from build123d import *

# Parameters (mm, degrees)
SKETCH1_R                   = 13.21
SKETCH1_R_2                 = 2.1
BOSS_EXTRUDE1_DEPTH         = 20
CHAMFER1_SIZE               = 1.2
BOSS_EXTRUDE5_START         = 40
SKETCH7_R                   = 13.21
SKETCH7_R_2                 = 3.3
BOSS_EXTRUDE5_DEPTH         = 40
CUT_EXTRUDE3_START          = -0.5
SKETCH8_W                   = 13.21
SKETCH8_H                   = 35.8
CUT_EXTRUDE3_DEPTH          = 1
SKETCH11_W                  = 13.21
SKETCH11_H                  = 35.8
CUT_EXTRUDE5_DEPTH          = 2.5
CUT_EXTRUDE6_DEPTH          = 45.29975395
CUT_EXTRUDE6_DEPTH_BACK     = 45.29975395
SKETCH12_R                  = 1.2
SKETCH13_R                  = 2.5
CUT_EXTRUDE7_DEPTH          = 47.093038676
SKETCH15_R                  = 1.8
BOSS_EXTRUDE6_DEPTH         = 5
BOSS_EXTRUDE7_REACH         = 61.49
CIRPATTERN2_COUNT           = 4
CIRPATTERN2_COPY_1_SKETCH_R = 1.8
CIRPATTERN2_COPY_1_DEPTH    = 5
CIRPATTERN2_COPY_2_SKETCH_R = 1.8
CIRPATTERN2_COPY_2_DEPTH    = 5
CIRPATTERN2_COPY_3_SKETCH_R = 1.8
CIRPATTERN2_COPY_3_DEPTH    = 5
CHAMFER2_SIZE               = 6.994614872
CHAMFER2_SIZE2              = 15


with BuildPart() as part:
    # Sketch1 → Boss-Extrude1 (new body)
    with BuildSketch(Plane(origin=(0, 0, 0), x_dir=(1, 0, 0), z_dir=(0, 1, 0))):
        with Locations(Location((0, 0, 0), (0, 0, 270))):
            Circle(SKETCH1_R)
        with Locations(Location((0, 0, 0), (0, 0, 270))):
            Circle(SKETCH1_R_2, mode=Mode.SUBTRACT)
    extrude(amount=BOSS_EXTRUDE1_DEPTH)

    # Chamfer1
    chamfer1_edges = [part.edges().sort_by_distance(p)[0] for p in [
        (0, 0, -2.1),
    ]]
    chamfer(chamfer1_edges, length=CHAMFER1_SIZE)

    # Sketch7 → Boss-Extrude5 (add)
    with BuildSketch(Plane.XZ.offset(BOSS_EXTRUDE5_START)):
        with Locations(Location((0, 0, 0), (0, 0, 270))):
            Circle(SKETCH7_R)
        with Locations(Location((0, 0, 0), (0, 0, 270))):
            Circle(SKETCH7_R_2, mode=Mode.SUBTRACT)
    extrude(amount=-BOSS_EXTRUDE5_DEPTH)

    # Sketch8 → Cut-Extrude3 (cut)
    with BuildSketch(Plane(origin=(0, 0, 0), x_dir=(0, 0, -1), z_dir=(1, 0, 0)).offset(CUT_EXTRUDE3_START)):
        with Locations((-6.605, -22.1)):
            Rectangle(SKETCH8_W, SKETCH8_H)
    extrude(amount=CUT_EXTRUDE3_DEPTH, mode=Mode.SUBTRACT)

    # Sketch11 → Cut-Extrude5 (cut, symmetric)
    with BuildSketch(Plane(origin=(0, 0, 0), x_dir=(0, 0, -1), z_dir=(1, 0, 0))):
        with Locations((6.605, -22.1)):
            Rectangle(SKETCH11_W, SKETCH11_H)
    extrude(amount=CUT_EXTRUDE5_DEPTH, both=True, mode=Mode.SUBTRACT)

    # Sketch12 → Cut-Extrude6 (cut, two sides: drawn at the far end of the back side and taken through both)
    with BuildSketch(Plane.ZY.offset(-0.5).offset(-CUT_EXTRUDE6_DEPTH_BACK)):
        with Locations((10.21, -8.2)):
            Circle(SKETCH12_R)
    extrude(amount=CUT_EXTRUDE6_DEPTH + CUT_EXTRUDE6_DEPTH_BACK, mode=Mode.SUBTRACT)

    # Sketch13 → Cut-Extrude7 (cut, through all)
    with BuildSketch(Plane.ZY.offset(-5.5)):
        with Locations((10.21, -8.2)):
            Circle(SKETCH13_R)
    cut_extrude7 = extrude(amount=-CUT_EXTRUDE7_DEPTH, mode=Mode.SUBTRACT)

    # Mirror2: Cut-Extrude7 across plane
    add(cut_extrude7.mirror(Plane(origin=(0, 0, 0), x_dir=(0, 0, 1), z_dir=(1, 0, 0))), mode=Mode.SUBTRACT)

    # Sketch15 → Boss-Extrude6 (add)
    with BuildSketch(Plane(origin=(-1.060660172, 0, -1.060660172), x_dir=(-0.7071067811865488, -3.372135297382167e-15, 0.7071067811865462), z_dir=(-0.7071067811865462, 3.3721352973821793e-15, -0.7071067811865488))):
        Polygon((-22.70423895, -23.81017386), (-11.21, -23.81017386), (-11.21, -35.211035784), (-11.21, -40), (-15.990174244, -46.657077484), (-29.831605047, -40.876524454), align=None)
        with Locations((-19.21, -29.81017386)):
            Circle(SKETCH15_R, mode=Mode.SUBTRACT)
        with Locations((-19.21, -38.81017386)):
            Circle(SKETCH15_R, mode=Mode.SUBTRACT)
    boss_extrude6 = extrude(amount=BOSS_EXTRUDE6_DEPTH)

    # Mirror3: Boss-Extrude6 across plane
    add(boss_extrude6.mirror(Plane(origin=(0, 0, 0), x_dir=(-0.7071067811865488, 3.3721352973821916e-15, 0.7071067811865464), z_dir=(0.7071067811865462, -3.3721352973821793e-15, 0.7071067811865488))))

    # Boss-Extrude7: up to this face of the body (flat: up to its plane)
    boss_extrude7_end = Plane(part.part.faces().sort_by_distance((18.066702505, -34.728946199, -8.87431435))[0])
    # Sketch16 → Boss-Extrude7 (add, up to the picked face)
    with BuildSketch(Plane(origin=(-4.596194078, 0, -4.596194078), x_dir=(-0.7071067811865486, -3.1363800445660566e-15, 0.7071067811865465), z_dir=(-0.7071067811865465, 3.1363800445660664e-15, -0.7071067811865486)), mode=Mode.PRIVATE) as boss_extrude7_sk1:
        with BuildLine():
            Line((-11.500178259, -23.81017386), (-22.70423895, -23.81017386))
            ThreePointArc((-22.70423895, -23.81017386), (-18.231146382, -18.383887076), (-11.500178259, -16.347416226))
            Line((-11.500178259, -16.347416226), (-11.500178259, -23.81017386))
        make_face()
    boss_extrude7_tool1 = split(extrude(boss_extrude7_sk1.sketch, amount=-BOSS_EXTRUDE7_REACH, mode=Mode.PRIVATE), bisect_by=boss_extrude7_end, keep=Keep.BOTH, mode=Mode.PRIVATE)
    boss_extrude7 = boss_extrude7_tool1.solids().sort_by(Axis((6.682248, -20.729124, -15.874636), (0.7071067811865465, -3.1363800445660664e-15, 0.7071067811865486)))[0]
    add(boss_extrude7)

    # CirPattern2: Boss-Extrude6, Boss-Extrude7 ×4 about axis
    cirpattern2_axis = Axis((0, 0, 0), (0, 1, 0))
    add([boss_extrude6.rotate(cirpattern2_axis, i * 360 / CIRPATTERN2_COUNT) for i in range(1, CIRPATTERN2_COUNT)])
    add([boss_extrude7.rotate(cirpattern2_axis, i * 360 / CIRPATTERN2_COUNT) for i in range(1, CIRPATTERN2_COUNT)])

    # CirPattern2 copy 1 sketch → CirPattern2 copy 1 (add)
    with BuildSketch(Plane(origin=(1.060660172, 0, -1.060660172), x_dir=(0.7071067811865462, -3.372135297382167e-15, 0.7071067811865489), z_dir=(0.7071067811865488, -3.3721352973821793e-15, -0.7071067811865461))):
        Polygon((-22.70423895, 23.81017386), (-11.21, 23.81017386), (-11.21, 35.211035784), (-11.21, 40), (-15.990174244, 46.657077484), (-29.831605047, 40.876524454), align=None)
        with Locations((-19.21, 29.81017386)):
            Circle(CIRPATTERN2_COPY_1_SKETCH_R, mode=Mode.SUBTRACT)
        with Locations((-19.21, 38.81017386)):
            Circle(CIRPATTERN2_COPY_1_SKETCH_R, mode=Mode.SUBTRACT)
    extrude(amount=CIRPATTERN2_COPY_1_DEPTH)

    # CirPattern2 copy 2 sketch → CirPattern2 copy 2 (add)
    with BuildSketch(Plane(origin=(-1.060660172, 0, -1.060660172), x_dir=(0.7071067811865489, -3.372135297382167e-15, -0.7071067811865462), z_dir=(-0.7071067811865461, -3.3721352973821793e-15, -0.7071067811865488))):
        Polygon((-22.70423895, 23.81017386), (-11.21, 23.81017386), (-11.21, 35.211035784), (-11.21, 40), (-15.990174244, 46.657077484), (-29.831605047, 40.876524454), align=None)
        with Locations((-19.21, 29.81017386)):
            Circle(CIRPATTERN2_COPY_2_SKETCH_R, mode=Mode.SUBTRACT)
        with Locations((-19.21, 38.81017386)):
            Circle(CIRPATTERN2_COPY_2_SKETCH_R, mode=Mode.SUBTRACT)
    extrude(amount=CIRPATTERN2_COPY_2_DEPTH)

    # CirPattern2 copy 3 sketch → CirPattern2 copy 3 (add)
    with BuildSketch(Plane(origin=(-1.060660172, 0, 1.060660172), x_dir=(-0.7071067811865461, -3.372135297382167e-15, -0.707106781186549), z_dir=(-0.7071067811865489, -3.3721352973821793e-15, 0.707106781186546))):
        Polygon((-22.70423895, 23.81017386), (-11.21, 23.81017386), (-11.21, 35.211035784), (-11.21, 40), (-15.990174244, 46.657077484), (-29.831605047, 40.876524454), align=None)
        with Locations((-19.21, 29.81017386)):
            Circle(CIRPATTERN2_COPY_3_SKETCH_R, mode=Mode.SUBTRACT)
        with Locations((-19.21, 38.81017386)):
            Circle(CIRPATTERN2_COPY_3_SKETCH_R, mode=Mode.SUBTRACT)
    extrude(amount=CIRPATTERN2_COPY_3_DEPTH)

    # Chamfer2
    chamfer2_edges = [part.edges().sort_by_distance(p)[0] for p in [
        (0, 20, -13.21),
    ]]
    chamfer2_side = [part.faces().sort_by_distance(p)[0] for p in [
        (0, 20, -12.836364777),
    ]]
    chamfer(chamfer2_edges, length=CHAMFER2_SIZE, length2=CHAMFER2_SIZE2, reference=chamfer2_side[0])


solid = part.part
Geometry check sheet. Reference: the model listing, model coordinates, mm. A direction names the side the tool comes from. Give positions to 0.01 mm unless a question says otherwise; leave off trailing zeros. Order: outer loops, then holes, each group sorted by start corner. A loop starts at its lowest first (then second) coordinate and runs counter-clockwise, first axis right, second up.
1) Material ranges on probe 1 along Z at (x, y) = (-9, -26); probe 2 along X at (y, z) = (-37.5, -10.5); probe 3 along X at (y, z) = (-29, -10.5), recorded low to high.
Results are:
probe 1: z = -18.19 to -11.12, -9.67 to 9.67, 11.12 to 18.19
probe 2: x = -19.69 to -18.41, -14.92 to -12.62, -8.38 to -2.5, 2.5 to 8.38, 12.62 to 14.92, 18.41 to 19.69
probe 3: x = -19.69 to -18.94, -14.39 to -12.62, -8.38 to -2.5, 2.5 to 8.38, 12.62 to 14.39, 18.94 to 19.69
2) Gauge pin test, flat ends, axial feed: pin 1 (12 mm diameter, centred on y = -17.5, z = 16, fed in from -X) (3 decimals); pin 2 (6.5 mm diameter, centred on x = 0, z = 0, fed in from +Y); pin 3 (1.9 mm diameter, centred on y = -8.2, z = 10.21, fed in from -X) (3 decimals); pin 4 (4.5 mm diameter, centred on y = -7, z = 11, fed in from -X). Record the tip position at first contact, or that the pin passes through.
Results are:
pin 1: stops at x = -18.785
pin 2: stops at y = 20
pin 3: passes through
pin 4: stops at x = -9.7
3) Tool access check on faces 4 (the cylindrical face through (-10.946, -31.595, -16.553)), 5 (the flat face through (13, -23.81, 13)). Record the directions out of +Z, -Z, +X, -X, +Y, -Y that give a thin tool (end or side, any length) a straight path to the whole face; none if there is none.
Results are:
face 4: none
face 5: -Y
4) Draft check along Z on faces 1 (the flat face through (21.41, -32.46, 15.81)), 2 (the cylindrical face through (-16.553, -40.595, 10.946)), 3 (the flat face through (-15.81, -32.46, -21.41)). Enter one of: released by +Z, released by -Z, zero draft, split by the parting line, or undercut.
Results are:
face 1: released by +Z
face 2: undercut
face 3: released by -Z
5) Cross-section at A-A (z = 0). Record the boundary of the cut face in (x, y).
Results are:
outline: (-13.21, -40) - (-3.3, -40) - (-3.3, 0) - (-2.1, 1.2) - (-2.1, 20) - (-6.22, 20) - (-13.21, 5) - close; (2.1, 1.2) - (3.3, 0) - (3.3, -40) - (13.21, -40) - (13.21, 5) - (6.22, 20) - (2.1, 20) - close
6) Cross-section at C-C (y = -38). Give the number of separate pieces and of enclosed holes in the cut face, then the cut area to 3 significant figures.
Results are:
separate pieces: 10
enclosed holes: 0
area: 970 mm2
7) Cross-section at B-B (y = 15). Record the boundary of the cut face in (x, z).
Results are:
outline: circle Ø17.09 at (0, 0); hole circle Ø4.2 at (0, 0)
